Autodesk Inventor part; units mm, degrees
ref_plane "YZ Plane" through (0, 0, 0) normal (1, 0, 0) x (0, 1, 0)
ref_plane "XZ Plane" through (0, 0, 0) normal (0, 1, 0) x (-1, 0, 0)
ref_plane "XY Plane" through (0, 0, 0) normal (0, 0, 1) x (1, 0, 0)
sketch "Sketch1" plane through (0, 0, 0) normal (0, 1, 0) x (-1, 0, 0)
  line L0 (23.8582, 45.9592) -> (-40.1418, 45.9592)
  line L1 (-40.1418, 45.9592) -> (-40.1418, -94.0408)
  line L2 (-40.1418, -94.0408) -> (23.8582, -94.0408)
  line L3 (23.8582, -94.0408) -> (23.8582, 45.9592)
  point P0 (0, 0)
  dimension "d0" = 140
  dimension "d1" = 64
extrude "Extrusion1" add sketch "Sketch1" along normal blind 36
sketch "Sketch2" plane through (40.1418, 0, 45.9592) normal (1, 0, 0) x (0, 0, -1)
  line L0 (0, 0) -> (140, 0)
  line L1 (0, 36) -> (140, 36)
  line L2 (0, 0) -> (0, 36)
  line L3 (140, 0) -> (0, 35)
  line L4 (0, 0) -> (0, 36)
  point P0 (45.9592, 0)
  dimension "d35" = 1
extrude "Extrusion2" cut sketch "Sketch2" against normal through all
sketch "Sketch5" plane through (40.1418, 36, -94.0408) normal (0, 0, -1) x (-1, 0, 0)
  line L0 (64, 0) -> (0, 0)
  line L1 (0, 0) -> (0, 35)
  line L2 (0, 35) -> (64, 35)
  line L3 (64, 35) -> (64, 0)
  line L4 (64, -36) -> (64, 0)
  line L5 (0, -36) -> (0, 0)
  line L6 (0, 0) -> (64, 0)
  point P0 (40.1418, -36)
  dimension "d18" = 0
  dimension "d19" = 0
  dimension "d20" = 35
  dimension "d23" = 0
extrude "Extrusion3" add sketch "Sketch5" against normal blind 140
sketch "Sketch8" plane through (40.1418, 0, -94.0408) normal (0, 0, -1) x (-1, 0, 0)
  circle A0 centre (32, 66) radius 30
  line L0 (0, 0) -> (64, 0)
  line L1 (0, 0) -> (0, 71)
  point P0 (40.1418, 0)
  dimension "d43" = 66
  dimension "d44" = 32
  dimension "d45" = 60
extrude "Extrusion6" cut sketch "Sketch8" against normal through all
sketch "Sketch9" plane through (-23.8582, 0, -94.0408) normal (-1, 0, 0) x (0, 0, 1)
  circle A0 centre (20, 68) radius 1.5
  circle A1 centre (120, 68) radius 1.5
  line L0 (0, 0) -> (0, 71)
  line L1 (0, 71) -> (140, 71)
  point P0 (94.0408, 0)
  dimension "d48" = 20
  dimension "d49" = 3
  dimension "d50" = 3
  dimension "d51" = 3
  dimension "d52" = 3
  dimension "d53" = 120
extrude "Extrusion7" cut sketch "Sketch9" against normal through all
sketch "Sketch10" plane through (-23.8582, 0, -94.0408) normal (-1, 0, 0) x (0, 0, 1)
  line L0 (140, 35) -> (140, 71)
  line L1 (140, 35) -> (131, 71)
  line L2 (0, 0) -> (140, 35)
  line L3 (140, 71) -> (131, 71)
  line L4 (0, 71) -> (140, 71)
  line L5 (140, 71) -> (0, 71)
  line L6 (12, 71) -> (12, 3)
  line L7 (0, 0) -> (0, 71)
  point P0 (94.0408, 0)
  dimension "d56" = 90
  dimension "d67" = 12
extrude "Extrusion8" cut sketch "Sketch10" against normal through all contours L1 L3 L0 | L2 L7 L4 L6
sketch "Sketch11" plane through (-23.8582, 0, -94.0408) normal (0, -0.9701, 0.2425) x (1, 0, 0)
  circle A0 centre (32, 124.3087) radius 1.5
  line L0 (0, 0) -> (0, 144.3087)
  line L1 (0, 144.3087) -> (64, 144.3087)
  circle A1 centre (32, 94.3087) radius 1.5
  point P0 (23.8582, 91.2329)
  dimension "d59" = 3
  dimension "d60" = 32
  dimension "d61" = 20
  dimension "d62" = 32
  dimension "d63" = 50
  dimension "d64" = 3
extrude "Extrusion9" cut sketch "Sketch11" against normal through all
properties part number "rampe-goulotte"
Source: CAD feature listing. Evaluate the final solid. Frame: model axes, mm. Round coordinates to 2 decimals unless told otherwise and drop trailing zeros. Loops run counter-clockwise (first coordinate to the right, second up) from the corner with the lowest first, then second, coordinate; pieces in that order, holes last.
1. Ray query, L1, parallel to Z at x = 39.1, y = 68; L2, parallel to X at y = 66.5, z = -36; L3, parallel to X at y = 67, z = -45. Return the intervals inside material, ascending.
2. Section query A-A on y = 52.5. Output: boundary loops of the cut face in (x, z), and give its area (3 significant figures).
3. Contact query for flat-ended pins moving along their axis: pin 1 (4 mm diameter, centred on x = 27, z = -14.5, fed in from +Y); pin 2 (8 mm diameter, centred on x = -2.5, z = 2.5, fed in from -Y); pin 3 (8 mm diameter, centred on x = 11.5, z = 4.5, fed in from +Y). Output: stop coordinate, or through.
4. Section query C-C on z = 2. Output: boundary loops of the cut face in (x, y).
5. Section query D-D on x = 18.5. Output: boundary loops of the cut face in (y, z).
6. Section query B-B on y = 68. Output: boundary loops of the cut face in (x, z), and give its area (3 significant figures).
7. Mould query, pull axis X, two halves, no side actions, for faces 1 (the cylindrical face through (8.87, 36.01, -19.04)), 2 (the cylindrical face through (39.02, 69.26, -73.23)), 3 (the flat face through (40.142, 44, -19)). Classes: released by +X, released by -X, zero draft, split by the parting line, or undercut.
Answers below:
1. L1: z = -82.04 to -75.54, -72.54 to 24.46, 27.46 to 37.71
1. L2: x = -23.86 to -21.85, 38.14 to 40.14
1. L3: x = -23.86 to -21.84, 38.13 to 40.14
2. outline: (-23.86, -82.04) - (-18.65, -82.04) - (-18.65, 41.58) - (-23.86, 41.58) - close; (34.93, -82.04) - (40.14, -82.04) - (40.14, 41.58) - (34.93, 41.58) - close
2. area: 1,290 mm2
3. pin 1: stops at y = 44.44
3. pin 2: stops at y = 23.14
3. pin 3: stops at y = 36.92
4. outline: (-23.86, 24.01) - (40.14, 24.01) - (40.14, 71) - (37.72, 71) arc R30 cw (long way) to (-21.44, 71) - (-23.86, 71) - close
5. outline: (3, -82.04) - (37.84, -82.04) - (37.84, 45.25) - (35, 45.96) - close
6. outline: (-23.86, -82.04) - (-21.79, -82.04) - (-21.79, -75.54) - (-23.86, -75.54) - close; (-23.86, -72.54) - (-21.79, -72.54) - (-21.79, 24.46) - (-23.86, 24.46) - close; (-23.86, 27.46) - (-21.79, 27.46) - (-21.79, 37.71) - (-23.86, 37.71) - close; (38.08, -82.04) - (40.14, -82.04) - (40.14, -75.54) - (38.08, -75.54) - close; (38.08, -72.54) - (40.14, -72.54) - (40.14, 24.46) - (38.08, 24.46) - close; (38.08, 27.46) - (40.14, 27.46) - (40.14, 37.71) - (38.08, 37.71) - close
6. area: 470 mm2
7. face 1: undercut
7. face 2: zero draft
7. face 3: released by +X
